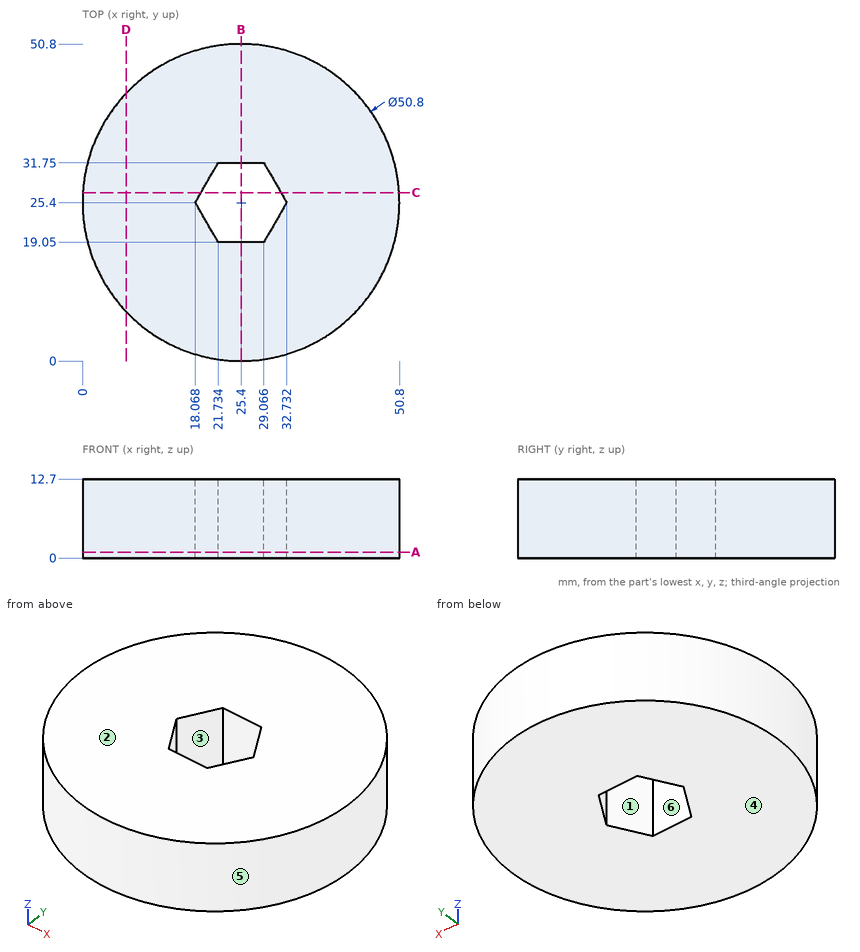
Verification items for this drawing (mm, ordinates from the low corner). A direction names the side the tool comes from. Give positions to 0.01 mm unless a question says otherwise; leave off trailing zeros. Write each loop counter-clockwise with the first axis right and the second up, starting at its lowest first coordinate (ties: lowest second). Pieces come first, ordered by that corner, then holes. Notation, with made-up numbers: (18.5, 64.25) - (36.5, 64.25) arc R23 cw to (36.5, 88.25) - close; hole circle Ø5 at (69.25, 47). An arc over 180 degrees is marked (long way). Answer as a JSON object with one key per item and string values. Group by question number.
1) Access from +Z, -Z, +X, -X, +Y, -Y to the whole of each face (thin tool, end or side, straight path). Record for the marked faces 1 and 2.
2) Sectioned sample at A-A (z = 1). Record the cut outline in (x, y), then the cut area to 3 significant figures.
3) Thickness scan on probe 1 along Y at (x, z) = (25, 4.75); probe 2 along Y at (x, z) = (30, 3) (1 decimal); probe 3 along X at (y, z) = (28, 2.5). Record the ranges inside material, lowest first. Write a range as from..to.
4) Sectioned sample at D-D (x = 7). Record the cut outline in (y, z).
5) Sectioned sample at C-C (y = 27). Record the cut outline in (x, z).
6) Sectioned sample at B-B (x = 25.4). Record the cut outline in (y, z).
7) Release check for a two-part mould opening along Y. For the marked faces 3, 4, 5 and 6 record: pulls with the +Y half, pulls with the -Y half, needs draft (parallel to the pull), parting line crosses it, or undercut.
8) Depth check by flat-ended pin: P1, Ø5, axis at y = 14, z = 8, coming from the -X side; P2, Ø4, axis at y = 6, z = 9, coming from the +X side (1 decimal); P3, Ø2, axis at x = 23.5, z = 4, coming from the +Y side. Enter the tip coordinate at first touch or a pass-through.
Geometry results:
{
 "1": {"face 1": "+Z, -Z", "face 2": "+Z, +X, -X, +Y, -Y"},
 "2": {"outline": "circle Ø50.8 at (25.4, 25.4); hole (18.07, 25.4) - (21.73, 19.05) - (29.07, 19.05) - (32.73, 25.4) - (29.07, 31.75) - (21.73, 31.75) - close", "area": "1,890 mm^2"},
 "3": {"probe 1": "y = 0..19.05, 31.75..50.8", "probe 2": "y = 0.4..20.7, 30.1..50.4", "probe 3": "x = 0.13..19.57, 31.23..50.67"},
 "4": {"outline": "(7.89, 0) - (42.91, 0) - (42.91, 12.7) - (7.89, 12.7) - close"},
 "5": {"outline": "(0.05, 0) - (18.99, 0) - (18.99, 12.7) - (0.05, 12.7) - close; (31.81, 0) - (50.75, 0) - (50.75, 12.7) - (31.81, 12.7) - close"},
 "6": {"outline": "(0, 0) - (19.05, 0) - (19.05, 12.7) - (0, 12.7) - close; (31.75, 0) - (50.8, 0) - (50.8, 12.7) - (31.75, 12.7) - close"},
 "7": {"face 3": "undercut", "face 4": "needs draft", "face 5": "parting line crosses it", "face 6": "undercut"},
 "8": {"P1": "stops at x = 1.61", "P2": "stops at x = 43.9", "P3": "stops at y = 50.78"}
}
